The model under review builds one solid part; all positions refer to its coordinate system, in mm. Face numbers are marked on the shaded views. A direction names the side the tool comes from. Round coordinates to 2 decimals unless told otherwise and drop trailing zeros. Loops run counter-clockwise (first coordinate to the right, second up) from the corner with the lowest first, then second, coordinate; pieces in that order, holes last. Notation, with made-up numbers: M 0.5,78.5 L 15.5,78.5 A27 ccw 15.5,100.5 Z; hole C 47.5,72 d4. An arc over 180 degrees is marked long. One line per question, with ' | ' between items.
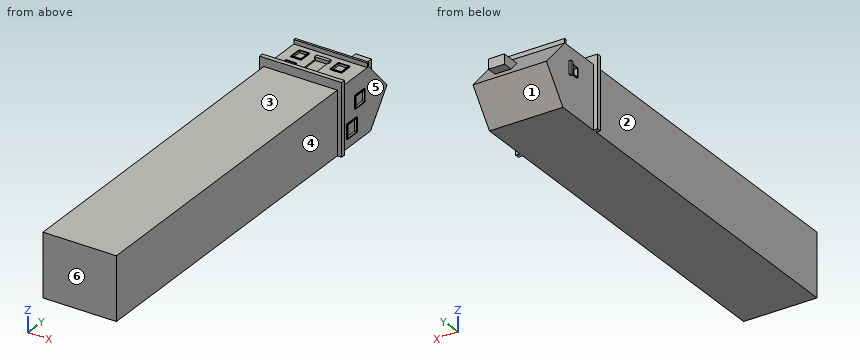
Autodesk Inventor part; units mm, degrees
ref_plane "工作平面1" through (8.5, 0, 0) normal (-1, 0, 0) x (0, 0, 1)
ref_plane "YZ Plane" through (0, 0, 0) normal (1, 0, 0) x (0, 1, 0)
ref_plane "XZ Plane" through (0, 0, 0) normal (0, 1, 0) x (-1, 0, 0)
sketch "草圖1" plane through (0, 0, 0) normal (1, 0, 0) x (0, 1, 0)
  line L0 (0, 0) -> (-6.4572, 7.1039)
  line L1 (-6.4572, 7.1039) -> (-6.4572, 8.1039)
  line L2 (-6.4572, 8.1039) -> (-6.9572, 8.1039)
  line L3 (-6.9572, 8.1039) -> (-6.9572, 7.1039)
  line L4 (-6.9572, 7.1039) -> (-16.5572, 7.1039)
  line L5 (-16.5572, 7.1039) -> (-16.5572, 9.1039)
  line L6 (-16.5572, 9.1039) -> (-17.5572, 9.1039)
  line L7 (-17.5572, 9.1039) -> (-17.5572, 0)
  line L8 (0, 0) -> (-5.811, -7.5155)
  line L9 (-5.811, -7.5155) -> (-17.5572, -7.5155)
  line L10 (-17.5572, -7.5155) -> (-17.5572, 0)
  dimension "d0" = 9.6
  dimension "d1" = 1
  dimension "d2" = 0.5
  dimension "d3" = 9.6
  dimension "d4" = 2
  dimension "d5" = 1
  dimension "d6" = 9.5
extrude "擠出1" add sketch "草圖1" along normal blind 17
sketch "草圖2" plane through (0, 0, 0) normal (-1, 0, 0) x (0, 0, 1)
  line L0 (1.3244, -10.5521) -> (3.3244, -10.5521)
  line L1 (3.3244, -10.5521) -> (3.3244, -8.5521)
  line L2 (3.3244, -8.5521) -> (1.3244, -8.5521)
  line L3 (1.3244, -8.5521) -> (1.3244, -10.5521)
  line L4 (1.3244, -10.5521) -> (3.3244, -8.5521) construction
  line L5 (3.3244, -10.5521) -> (1.3244, -8.5521) construction
  line L6 (0.8244, -8.5521) -> (3.8244, -8.5521)
  line L7 (3.8244, -8.5521) -> (3.8244, -7.9272)
  line L8 (3.8244, -7.9272) -> (0.8244, -7.9272)
  line L9 (0.8244, -7.9272) -> (0.8244, -8.5521)
  line L10 (1.2244, -10.6521) -> (3.4244, -10.6521)
  line L11 (3.4244, -10.6521) -> (3.4244, -8.4521)
  line L12 (3.4244, -8.4521) -> (1.2244, -8.4521)
  line L13 (1.2244, -8.4521) -> (1.2244, -10.6521)
  line L14 (1.2244, -10.6521) -> (3.4244, -8.4521) construction
  line L15 (3.4244, -10.6521) -> (1.2244, -8.4521) construction
  point P0 (0, 0)
  point P1 (2.3244, -9.5521)
  point P2 (0.8244, -8.2396)
  point P3 (1.2244, -8.5521)
  point P4 (3.4244, -8.5521)
  dimension "d9" = 0.5
  dimension "d10" = 0.5
  dimension "d15" = 0.1
  dimension "d16" = 0.1
  dimension "d17" = 0.1
  dimension "d18" = 0.1
  dimension "d19" = 2
extrude "擠出2" add sketch "草圖2" along normal blind 0.5 contours L6 L13 L12 L11 L2 | L6 L9 L8 L7 L11 L12 L13
extrude "擠出3" cut sketch "草圖2" against normal blind 0.5 contours L3 L2 L1 L0
extrude "擠出4" add sketch "草圖2" along normal blind 0.3 contours L0 L1 L6 L11 L10 L13 L3
sketch "草圖3" plane through (0, -16.5572, 7.1039) normal (0, 0, 1) x (1, 0, 0)
  line L0 (2.4891, 7.7612) -> (4.5073, 7.7612)
  line L1 (4.5073, 7.7612) -> (4.5073, 5.2048)
  line L2 (4.5073, 5.2048) -> (2.4891, 5.2048)
  line L3 (2.4891, 5.2048) -> (2.4891, 7.7612)
  line L4 (0, 0) -> (17, 0)
  line L5 (2.4891, 0) -> (4.5073, 0)
  line L6 (4.5073, 0) -> (4.5073, 3.1193)
  line L7 (4.5073, 3.1193) -> (2.4891, 3.1193)
  line L8 (2.4891, 3.1193) -> (2.4891, 0)
  line L9 (6.761, 6.8866) -> (9.6873, 6.8866)
  line L10 (9.6873, 6.8866) -> (9.6873, 2.6148)
  line L11 (9.6873, 2.6148) -> (6.761, 2.6148)
  line L12 (6.761, 2.6148) -> (6.761, 6.8866)
  line L13 (11.6046, 7.7612) -> (13.8583, 7.7612)
  line L14 (13.8583, 7.7612) -> (13.8583, 5.2048)
  line L15 (13.8583, 5.2048) -> (11.6046, 5.2048)
  line L16 (11.6046, 5.2048) -> (11.6046, 7.7612)
  point P0 (0, 16.5572)
extrude "擠出5" cut sketch "草圖3" against normal blind 0.3
sketch "草圖4" plane through (0, -16.5572, 7.1039) normal (0, 0, 1) x (1, 0, 0)
  line L0 (0, 0) -> (17, 0)
  line L1 (2.2891, 0) -> (4.7073, 0)
  line L2 (4.7073, 0) -> (4.7073, 3.3193)
  line L3 (4.7073, 3.3193) -> (2.2891, 3.3193)
  line L4 (2.2891, 3.3193) -> (2.2891, 0)
  line L5 (6.561, 6.8866) -> (9.8873, 6.8866)
  line L6 (9.8873, 6.8866) -> (9.8873, 7.667)
  line L7 (9.8873, 7.667) -> (6.561, 7.667)
  line L8 (6.561, 7.667) -> (6.561, 6.8866)
  line L9 (6.761, 2.6148) -> (6.761, 6.8866)
  line L10 (9.6873, 6.8866) -> (9.6873, 2.6148)
  line L11 (4.5073, 3.1193) -> (4.5073, 0)
  line L12 (2.4891, 0) -> (2.4891, 3.1193)
  line L13 (2.4891, 3.1193) -> (4.5073, 3.1193)
  line L14 (2.2891, 7.9612) -> (4.7073, 7.9612)
  line L15 (4.7073, 7.9612) -> (4.7073, 5.0048)
  line L16 (4.7073, 5.0048) -> (2.2891, 5.0048)
  line L17 (2.2891, 5.0048) -> (2.2891, 7.9612)
  line L18 (11.4046, 7.9612) -> (14.0583, 7.9612)
  line L19 (14.0583, 7.9612) -> (14.0583, 5.0048)
  line L20 (14.0583, 5.0048) -> (11.4046, 5.0048)
  line L21 (11.4046, 5.0048) -> (11.4046, 7.9612)
  line L22 (11.6046, 7.7612) -> (13.8583, 7.7612)
  line L23 (13.8583, 7.7612) -> (13.8583, 5.2048)
  line L24 (11.6046, 5.2048) -> (11.6046, 7.7612)
  line L25 (13.8583, 5.2048) -> (11.6046, 5.2048)
  line L26 (4.5073, 7.7612) -> (4.5073, 5.2048)
  line L27 (4.5073, 5.2048) -> (2.4891, 5.2048)
  line L28 (2.4891, 5.2048) -> (2.4891, 7.7612)
  line L29 (2.4891, 7.7612) -> (4.5073, 7.7612)
  line L30 (4.5073, 7.7612) -> (4.5073, 5.2048)
  line L31 (4.5073, 5.2048) -> (2.4891, 5.2048)
  line L32 (2.4891, 5.2048) -> (2.4891, 7.7612)
  line L33 (2.4891, 3.1193) -> (4.5073, 3.1193)
  line L34 (4.5073, 3.1193) -> (4.5073, 0)
  line L35 (4.5073, 0) -> (2.4891, 0)
  line L36 (2.4891, 0) -> (2.4891, 3.1193)
  line L37 (11.6046, 7.7612) -> (13.8583, 7.7612)
  line L38 (13.8583, 7.7612) -> (13.8583, 5.2048)
  line L39 (13.8583, 5.2048) -> (11.6046, 5.2048)
  line L40 (11.6046, 5.2048) -> (11.6046, 7.7612)
  point P0 (0, 16.5572)
  dimension "d24" = 0.2
  dimension "d25" = 0.2
  dimension "d26" = 0.2
  dimension "d27" = 0.2
  dimension "d28" = 0.2
  dimension "d29" = 0.2
  dimension "d30" = 0.2
  dimension "d31" = 0.2
  dimension "d32" = 0.2
  dimension "d33" = 0.2
  dimension "d34" = 0.2
  dimension "d35" = 0.2
extrude "擠出6" add sketch "草圖4" along normal blind 0.2 contours L4 L3 L2 L0 L11 L13 L12 | L14 L15 L16 L17 | L18 L19 L20 L21
extrude "擠出7" add sketch "草圖4" along normal blind 0.5 contours L8 L7 L6 L5
sketch "草圖5" plane through (17, 0, 0) normal (1, 0, 0) x (0, 0, -1)
  line L0 (-2.8354, -8.2564) -> (-0.2487, -8.2564)
  line L1 (-0.2487, -8.2564) -> (-0.2487, -11.3114)
  line L2 (-0.2487, -11.3114) -> (-2.8354, -11.3114)
  line L3 (-2.8354, -11.3114) -> (-2.8354, -8.2564)
  line L4 (2.2042, -10.9992) -> (5.1699, -10.9992)
  line L5 (5.1699, -10.9992) -> (5.1699, -14.1433)
  line L6 (5.1699, -14.1433) -> (2.2042, -14.1433)
  line L7 (2.2042, -14.1433) -> (2.2042, -10.9992)
  line L8 (-3.0354, -8.0564) -> (-0.0487, -8.0564)
  line L9 (-0.0487, -8.0564) -> (-0.0487, -11.5114)
  line L10 (-0.0487, -11.5114) -> (-3.0354, -11.5114)
  line L11 (-3.0354, -11.5114) -> (-3.0354, -8.0564)
  line L12 (2.0042, -10.7992) -> (5.3699, -10.7992)
  line L13 (5.3699, -10.7992) -> (5.3699, -14.3433)
  line L14 (5.3699, -14.3433) -> (2.0042, -14.3433)
  line L15 (2.0042, -14.3433) -> (2.0042, -10.7992)
  point P0 (0, 0)
  dimension "d40" = 0.2
  dimension "d41" = 0.2
  dimension "d42" = 0.2
  dimension "d43" = 0.2
  dimension "d44" = 0.2
  dimension "d45" = 0.2
  dimension "d46" = 0.2
  dimension "d47" = 0.2
extrude "擠出8" cut sketch "草圖5" against normal blind 0.3 contours L0 L1 L2 L3 | L4 L5 L6 L7
extrude "擠出9" add sketch "草圖5" along normal blind 0.2
sketch "草圖6" plane through (0, -17.5572, -7.5155) normal (0, -1, 0) x (1, 0, 0)
  line L0 (0, 0) -> (0, 7.5155)
  line L1 (17, 7.5155) -> (17, 14.6194)
  line L2 (0, 0) -> (17, 0)
  line L3 (17, 0) -> (17, 14.6194)
  line L4 (17, 14.6194) -> (0, 14.6194)
  line L5 (0, 14.6194) -> (0, 0)
extrude "擠出10" add sketch "草圖6" along normal blind 78
sketch "草圖7" plane through (0, 0, 0) normal (-1, 0, 0) x (0, 0, 1)
  line L0 (9.1039, -16.5572) -> (9.1039, -17.5572)
  line L1 (-7.5155, -5.811) -> (-7.5155, -95.5572)
  line L2 (9.1039, -17.5572) -> (-7.5155, -17.5572)
  line L3 (-7.5155, -17.5572) -> (-7.5155, -16.5572)
  line L4 (-7.5155, -16.5572) -> (9.1039, -16.5572)
  line L5 (9.1039, -16.5572) -> (9.1039, -17.5572)
  point P0 (0, 0)
  point P1 (-7.5155, -17.5572)
  dimension "d54" = 1
extrude "擠出11" add sketch "草圖7" along normal blind 1
ref_plane "工作平面1" through (8.5, 0, 0) normal (-1, 0, 0) x (0, 0, 1)
mirror "鏡射1" about plane through (8.5, 0, 0) normal (-1, 0, 0) of "擠出11"
sketch "草圖8" plane through (0, -17.5572, 7.1039) normal (0, -1, 0) x (1, 0, 0)
  line L0 (9.431, -2.7696) -> (13.1296, -2.7696)
  line L1 (13.1296, -2.7696) -> (13.1296, -5.0596)
  line L2 (13.1296, -5.0596) -> (9.431, -5.0596)
  line L3 (9.431, -5.0596) -> (9.431, -2.7696)
  point P0 (0, -7.1039)
extrude "擠出12" add sketch "草圖8" against normal blind 18
properties part number "屋1 物3"
1) Mouldability with a two-part tool opening along Y and no side actions: class the marked faces 4, 5 and 6 as +Y half, -Y half, draft (parallel to the pull), parting line (faces both ways), or undercut.
Output values:
face 4: draft | face 5: undercut | face 6: -Y half
2) Machinability: for the marked faces 1, 2 and 3, which of the approach directions +Z, -Z, +X, -X, +Y, -Y give a long, thin tool a straight path to every point of the face, cutting with its end or side? Answer none if there is none.
Output values:
face 1: -Z, +X, -X, +Y | face 2: +Z, -Z, -X, -Y | face 3: +Z, +X, -X, -Y
3) For line 1 (Y direction, x = 2, z = 7.25); line 2 (X direction, y = -42, z = 3.75); line 3 (Z direction, x = 6.5, y = -7), list the stretches that pass through material, from the lowest coordinate up.
Output values:
line 1: y = -17.56 to -16.56, -6.96 to -6.46 | line 2: x = 0 to 17 | line 3: z = -7.52 to 7.1
4) Add section A-A on y = -46.5. State the section outline as (x, z) points.
Output values:
outline: M 0,-7.52 L 17,-7.52 L 17,7.1 L 0,7.1 Z
5) Insertion check: P1, Ø10, axis at x = 14.5, y = -85.5, coming from the +Z side; P2, Ø0.6, axis at y = -9, z = 2, coming from the -X side; P3, Ø2.5, axis at x = 12, y = -10.5, coming from the +Z side. Each pin has a flat end and moves straight along its axis. Give the tip position at first contact, or say it passes through.
Output values:
P1: stops at z = 7.1 | P2: stops at x = 0.5 | P3: stops at z = 7.3
